from build123d import *

# Parameters (mm, degrees)
BOSS_EXTRUDE1_DEPTH            = 47.625
BOSS_EXTRUDE1_DEPTH_BACK       = 47.625
CHAMFER1_SIZE                  = 0.05
TAP_DRILL_FOR_10_32_TAP2_D     = 4.0386
TAP_DRILL_FOR_10_32_TAP2_DEPTH = 15.875
TAP_DRILL_FOR_10_32_TAP2_TIP   = 1.213317848
TAP_DRILL_FOR_10_32_TAP1_D     = 4.0386
TAP_DRILL_FOR_10_32_TAP1_DEPTH = 9.525
TAP_DRILL_FOR_10_32_TAP1_TIP   = 1.213317848


with BuildPart() as part:
    # Sketch3 → Boss-Extrude1 (new, two sides: drawn at the far end of the back side and taken through both)
    with BuildSketch(Plane.XY.offset(-BOSS_EXTRUDE1_DEPTH_BACK)):
        with BuildLine():
            Line((-1.5, 2.969696007), (-1.5, 4.769696007))
            ThreePointArc((-1.5, 4.769696007), (0, -5), (1.5, 4.769696007))
            Line((1.5, 4.769696007), (1.5, 2.969696007))
            Line((1.5, 2.969696007), (-1.5, 2.969696007))
        make_face()
    extrude(amount=BOSS_EXTRUDE1_DEPTH + BOSS_EXTRUDE1_DEPTH_BACK)

    # Chamfer1
    chamfer1_edges = [part.edges().sort_by_distance(p)[0] for p in [
        (0, -5, -47.625),
        (0, -5, 47.625),
    ]]
    chamfer(chamfer1_edges, length=CHAMFER1_SIZE)

    # Tap Drill for #10-32 Tap2
    with Locations(Plane(origin=(0, 0, -47.625), x_dir=(-1, 0, 0), z_dir=(0, 0, -1))):
        with Locations((0, 0)):
            Hole(TAP_DRILL_FOR_10_32_TAP2_D / 2, depth=TAP_DRILL_FOR_10_32_TAP2_DEPTH)
            with Locations((0, 0, -(TAP_DRILL_FOR_10_32_TAP2_DEPTH + TAP_DRILL_FOR_10_32_TAP2_TIP / 2))):  # 118° drill point
                Cone(0, TAP_DRILL_FOR_10_32_TAP2_D / 2, TAP_DRILL_FOR_10_32_TAP2_TIP, mode=Mode.SUBTRACT)

    # Tap Drill for #10-32 Tap1
    with Locations(Plane.XY.offset(47.625)):
        with Locations((0, 0)):
            Hole(TAP_DRILL_FOR_10_32_TAP1_D / 2, depth=TAP_DRILL_FOR_10_32_TAP1_DEPTH)
            with Locations((0, 0, -(TAP_DRILL_FOR_10_32_TAP1_DEPTH + TAP_DRILL_FOR_10_32_TAP1_TIP / 2))):  # 118° drill point
                Cone(0, TAP_DRILL_FOR_10_32_TAP1_D / 2, TAP_DRILL_FOR_10_32_TAP1_TIP, mode=Mode.SUBTRACT)


solid = part.part
The model under review builds one solid part; all positions refer to its coordinate system, in mm. A direction names the side the tool comes from. Coordinates: 2 decimals unless noted, no trailing zeros. Write each loop counter-clockwise with the first axis right and the second up, starting at its lowest first coordinate (ties: lowest second). Pieces come first, ordered by that corner, then holes. Notation, with made-up numbers: (67.25, 43.5) - (87.25, 43.5) arc R30 cw to (87.25, 81.5) - close; hole circle Ø1 at (76, 27.5). An arc over 180 degrees is marked (long way). Answer as CSV lines item,"result".
(1) Tool access review of faces 4 (the flat face through (1.5, 4, -1)), 5 (the cylindrical face through (-1.926, 0.607, 42.796)), 6 (the cylindrical face through (1.926, 0.607, -39.576)): name each direction out of +Z, -Z, +X, -X, +Y, -Y from which nothing blocks a thin tool from reaching the whole face with its end or side.
Data:
face 4,"+Z, -Z, +Y"
face 5,"+Z"
face 6,"-Z"
(2) Clearance check with flat-ended pins moving along their axes: pin 1 Ø1.5 at (y, z) = (2.5, 11.5) entering from -X; pin 2 Ø2 at (y, z) = (4, -0.5) entering from -X; pin 3 Ø1.5 at (x, z) = (-0.5, -17.5) entering from +Y. State where each tip first meets the part, or that it passes through.
Data:
pin 1,"stops at x = -4.68"
pin 2,"stops at x = -4"
pin 3,"stops at y = 2.97"
(3) Mouldability with a two-part tool opening along X and no side actions: class faces 1 (the cylindrical face through (0, -5, -1)), 2 (the conical face through (0.076, -0.342, -30.747)), 3 (the flat face through (-0.1, -2.2, -47.625)) as pulls with the +X half, pulls with the -X half, needs draft (parallel to the pull), parting line crosses it, or undercut.
Data:
face 1,"parting line crosses it"
face 2,"undercut"
face 3,"needs draft"
(4) For line 1 along Y through (x, z) = (0, 45); line 2 along X through (y, z) = (0, 44); line 3 along Y through (x, z) = (0, 13), list the stretches that pass through material, from the lowest coordinate up. Write a range as [from, to].
Data:
line 1,"y = [-5, -2.02], [2.02, 2.97]"
line 2,"x = [-5, -2.02], [2.02, 5]"
line 3,"y = [-5, 2.97]"
(5) We need section A-A (z = -12). Give the boundary of the cut face in (x, y).
Data:
outline,"(-1.5, 2.97) - (-1.5, 4.77) arc R5 ccw (long way) to (1.5, 4.77) - (1.5, 2.97) - close"
